Source: three-view drawing plus pictorial views. Frame: mm from the lowest corner of the part. Give positions to 0.01 mm unless a question says otherwise; leave off trailing zeros. Loops run counter-clockwise (first coordinate to the right, second up) from the corner with the lowest first, then second, coordinate; pieces in that order, holes last. Notation, with made-up numbers: M -7.5,80.5 L 49.5,80.5 A12 ccw 49.5,95.5 Z; hole C -4.75,88.25 d6. An arc over 180 degrees is marked long. One line per item, written item: value. Start each with the question number.
(1) Section B-B on x = 16.5. Output: boundary loops of the cut face in (y, z), plus the area to 3 significant figures.
(2) Section A-A on z = 12.5. Output: boundary loops of the cut face in (x, y).
(3) Section D-D on z = 22.75. Output: boundary loops of the cut face in (x, y), plus the area to 3 significant figures.
(4) Pin query (flat end, axial travel): P1, Ø1.5, axis at y = 25, z = 22, coming from the +X side. Return the tip coordinate at first contact, or that it passes through.
(5) Ray query, line 1 along Y through (x, z) = (4, 19); line 2 along Y through (x, z) = (28, 10.5); line 3 along Z through (x, y) = (16.5, 5.25). Return the intervals inside material, ascending. Write a range as from..to.
(6) Section C-C on y = 23.5. Output: boundary loops of the cut face in (x, z).
(7) Pull-direction query (Z, two-part tool) for the marked faces 1, 2 and 3; classes: released by +Z, released by -Z, zero draft, split by the parting line, or undercut.
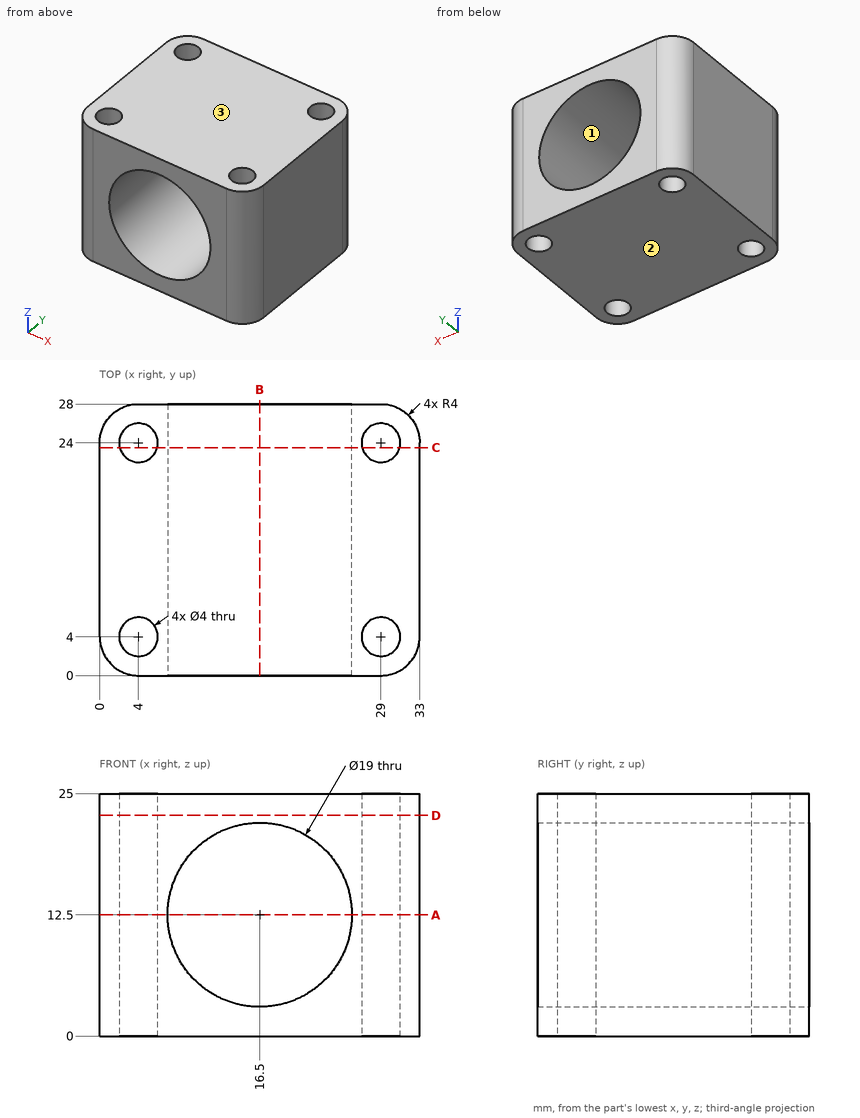
Output values:
1. outline: M 0,0 L 28,0 L 28,3 L 0,3 Z; M 0,22 L 28,22 L 28,25 L 0,25 Z
1. area: 168 mm²
2. outline: M 0,4 A4 ccw 4,0 L 7,0 L 7,28 L 4,28 A4 ccw 0,24 Z; M 26,0 L 29,0 A4 ccw 33,4 L 33,24 A4 ccw 29,28 L 26,28 Z; hole C 4,4 d4; hole C 4,24 d4; hole C 29,4 d4; hole C 29,24 d4
3. outline: M 0,4 A4 ccw 4,0 L 29,0 A4 ccw 33,4 L 33,24 A4 ccw 29,28 L 4,28 A4 ccw 0,24 Z; hole C 4,4 d4; hole C 4,24 d4; hole C 29,4 d4; hole C 29,24 d4
3. area: 860 mm²
4. P1: stops at x = 32.99
5. line 1: y = 0..2, 6..22, 26..28
5. line 2: y = 0..2.27, 5.73..22.27, 25.73..28
5. line 3: z = 0..3, 22..25
6. outline: M 0,0 L 2.06,0 L 2.06,25 L 0,25 Z; M 5.94,0 L 27.06,0 L 27.06,25 L 5.94,25 Z; M 30.94,0 L 33,0 L 33,25 L 30.94,25 Z; hole C 16.5,12.5 d19
7. face 1: undercut
7. face 2: released by -Z
7. face 3: released by +Z
